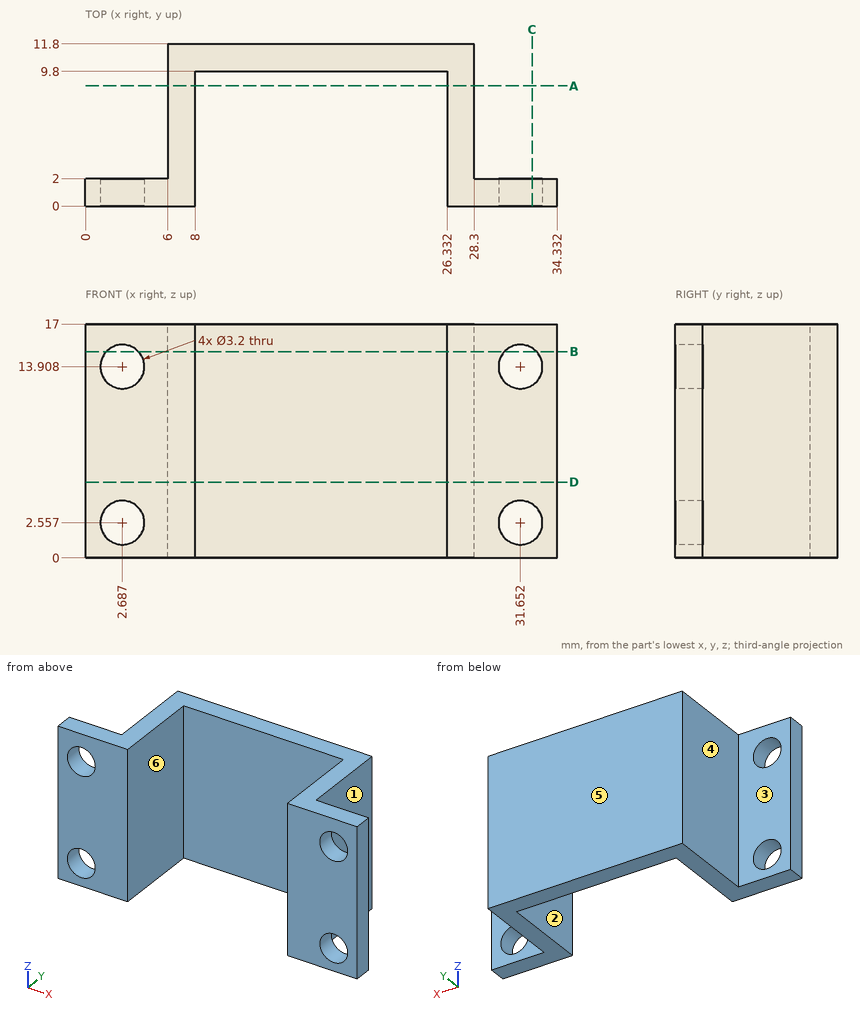
For this review, use the dimensioned drawing (mm, ordinates from the lowest corner) and the shaded views. A direction names the side the tool comes from. Coordinates: 2 decimals unless noted, no trailing zeros. Order: outer loops, then holes, each group sorted by start corner. A loop starts at its lowest first (then second) coordinate and runs counter-clockwise, first axis right, second up. Notation, with made-up numbers: M 21,19.25 L 73,19.25 A20 ccw 73,55.25 Z; hole C 7.25,-32.75 d1. An arc over 180 degrees is marked long. Answer as a JSON object with one key per item and string values. Group by question number.
1) Wall thickness on L1, parallel to X at y = 3.5, z = 13.75; L2, parallel to Y at x = 8.5, z = 12; L3, parallel to Y at x = 2, z = 8.25: over which ranges is each line inside the solid? List them lowest first.
2) Mouldability with a two-part tool opening along X and no side actions: class the marked faces 4, 5 and 6 as pulls with the +X half, pulls with the -X half, needs draft (parallel to the pull), parting line crosses it, or undercut.
3) Add section A-A, the plane y = 8.75. Write out the cut boundary in (x, z).
4) Add section C-C, the plane x = 32.5. Write out the cut boundary in (y, z) (1 decimal).
5) Add section D-D, the plane z = 5.5. Write out the cut boundary in (x, y).
6) Add section B-B, the plane z = 15. Write out the cut boundary in (x, y) (1 decimal).
7) For pin 1 (4 mm diameter, centred on x = 5, z = 10, fed in from -Y); pin 2 (3.5 mm diameter, centred on x = 31.65, z = 2.56, fed in from +Y); pin 3 (5 mm diameter, centred on y = 7, z = 9, fed in from +X); pin 4 (3 mm diameter, centred on x = 2.69, z = 2.56, fed in from +Y), all flat-tipped, find the tip position at first contact; note any pin that passes through.
8) Tool access review of the marked faces 1, 2 and 3: name each direction out of +Z, -Z, +X, -X, +Y, -Y from which nothing blocks a thin tool from reaching the whole face with its end or side.
Computed values:
{
 "1": {"L1": "x = 6 to 8, 26.33 to 28.3", "L2": "y = 9.8 to 11.8", "L3": "y = 0 to 2"},
 "2": {"face 4": "pulls with the -X half", "face 5": "needs draft", "face 6": "undercut"},
 "3": {"outline": "M 6,0 L 8,0 L 8,17 L 6,17 Z; M 26.33,0 L 28.3,0 L 28.3,17 L 26.33,17 Z"},
 "4": {"outline": "M 0,0 L 2,0 L 2,1.2 L 0,1.2 Z; M 0,3.9 L 2,3.9 L 2,12.6 L 0,12.6 Z; M 0,15.3 L 2,15.3 L 2,17 L 0,17 Z"},
 "5": {"outline": "M 0,0 L 8,0 L 8,9.8 L 26.33,9.8 L 26.33,0 L 34.33,0 L 34.33,2 L 28.3,2 L 28.3,11.8 L 6,11.8 L 6,2 L 0,2 Z"},
 "6": {"outline": "M 0,0 L 1.5,0 L 1.5,2 L 0,2 Z; M 3.9,0 L 8,0 L 8,9.8 L 26.3,9.8 L 26.3,0 L 30.5,0 L 30.5,2 L 28.3,2 L 28.3,11.8 L 6,11.8 L 6,2 L 3.9,2 Z; M 32.8,0 L 34.3,0 L 34.3,2 L 32.8,2 Z"},
 "7": {"pin 1": "stops at y = 0", "pin 2": "stops at y = 2", "pin 3": "stops at x = 28.3", "pin 4": "passes through"},
 "8": {"face 1": "+Z, -Z, +X, +Y", "face 2": "+Z, -Z, -Y", "face 3": "+Z, -Z, -X, +Y"}
}
